The listing builds one solid part. Answer for the finished solid, in the listing's coordinates (mm). A direction names the side the tool comes from. Round coordinates to 2 decimals unless told otherwise and drop trailing zeros. Write each loop counter-clockwise with the first axis right and the second up, starting at its lowest first coordinate (ties: lowest second). Pieces come first, ordered by that corner, then holes. Notation, with made-up numbers: M 71,37.25 L 77,37.25 A9 ccw 77,50.25 Z; hole C 49,-17.75 d10. An arc over 180 degrees is marked long. One line per item, written item: value. Start each with the question number.
(1) Given P1, Ø4, axis at y = 17, z = 5.5, coming from the -X side; P2, Ø10, axis at x = 26.5, y = 15, coming from the +Z side; P3, Ø3, axis at y = -1, z = 7, coming from the +X side, each flat-ended and moving along its own axis, determine where each tip first touches the part or whether it passes through.
(2) Section D-D (y = 2.5) is taken. Determine the outline of the cut face in (x, z).
(3) For a pull along Y with two mould halves and no side action, classify faces 1 (the flat face through (37.465, 12.773, 7.395)), 2 (the flat face through (31, 11, 15)), 3 (the flat face through (30, 12, 7)), 4 (the cylindrical face through (0.9, -0.86, 7.6)) as released by +Y, released by -Y, zero draft, split by the parting line, or undercut.
(4) Section C-C (y = 18.5) is taken. Determine the outline of the cut face in (x, z).
(5) For faces 5 (the cylindrical face through (1.252, -2.614, 0.562)), 6 (the flat face through (16, 0, 7)), determine the directions among +Z, -Z, +X, -X, +Y, -Y from which every point of the face is accessible in a straight line to the end or side of a thin tool.
(6) Section B-B (z = 8.75) is taken. Determine the outline of the cut face in (x, y).
(7) Section A-A (x = 12.5) is taken. Determine the outline of the cut face in (y, z), plus the area to 3 significant figures.
(8) Consider probe 1 along Y at (x, z) = (3, 9.5); probe 2 along Y at (x, z) = (31, 12.25); probe 3 along X at (y, z) = (29, 9.5). Determine where each line is inside the solid, lowest interval first.
```python
from build123d import *

# Parameters (mm, degrees)
PAD_DEPTH   = 15
FILLET_R    = 3
FILLET001_R = 0.5


with BuildPart() as part:
    # Sketch → Pad (new body)
    with BuildSketch(Plane.XY):
        Polygon((0, 0), (30, 0), (30, 25), (0, 25), (0, 32), (35, 32), (40, -7), (0, -7), align=None)
    extrude(amount=PAD_DEPTH)

    # Fillet
    fillet_edges = [part.edges().sort_by_distance(p)[0] for p in [
        (17.5, 32, 15),
        (17.5, 32, 0),
        (0, 32, 7.5),
        (0, 25, 7.5),
        (0, 28.5, 0),
        (0, 28.5, 15),
        (0, 0, 7.5),
        (0, -3.5, 0),
        (0, -7, 7.5),
        (0, -3.5, 15),
        (20, -7, 15),
        (20, -7, 0),
    ]]
    fillet(fillet_edges, radius=FILLET_R)

    # Fillet001
    fillet001_edges = [part.edges().sort_by_distance(p)[0] for p in [
        (16.5, 0, 15),
        (16.5, 0, 0),
        (16.5, 25, 0),
        (16.5, 25, 15),
        (30, 12.5, 0),
        (30, 12.5, 15),
    ]]
    fillet(fillet001_edges, radius=FILLET001_R)


solid = part.part
```
Recorded:
1. P1: stops at x = 30
1. P2: stops at z = 15
1. P3: stops at x = 39.42
2. outline: M 30,0.5 A0.5 ccw 30.5,0 L 38.78,0 L 38.78,15 L 30.5,15 A0.5 ccw 30,14.5 Z
3. face 1: released by +Y
3. face 2: zero draft
3. face 3: undercut
3. face 4: undercut
4. outline: M 30,0.5 A0.5 ccw 30.5,0 L 36.73,0 L 36.73,15 L 30.5,15 A0.5 ccw 30,14.5 Z
5. face 5: -Z, -X, +Y, -Y
5. face 6: +Z, -Z, -X
6. outline: M 0,-4 A3 ccw 3,-7 L 40,-7 L 35,32 L 3,32 A3 ccw 0,29 L 0,28 A3 ccw 3,25 L 30,25 L 30,0 L 3,0 A3 ccw 0,-3 Z
7. outline: M -7,3 A3 ccw -4,0 L -0.5,0 A0.5 ccw 0,0.5 L 0,14.5 A0.5 ccw -0.5,15 L -4,15 A3 ccw -7,12 Z; M 25,0.5 A0.5 ccw 25.5,0 L 29,0 A3 ccw 32,3 L 32,12 A3 ccw 29,15 L 25.5,15 A0.5 ccw 25,14.5 Z
7. area: 202 mm2
8. probe 1: y = -7 to 0, 25 to 32
8. probe 2: y = -6.99 to 31.99
8. probe 3: x = 0 to 35.38
